Read the model definition and answer for the solid it produces. Units are mm, in the model's axes. A direction names the side the tool comes from. Round coordinates to 2 decimals unless told otherwise and drop trailing zeros. Write each loop counter-clockwise with the first axis right and the second up, starting at its lowest first coordinate (ties: lowest second). Pieces come first, ordered by that corner, then holes. Notation, with made-up numbers: (51, 62) - (87, 62) arc R21 cw to (87, 80) - close; hole circle Ø5 at (-9, 51). An arc over 180 degrees is marked (long way). Answer as CSV lines item,"result". Start each with the question number.
1) Find section A-A on z = 15.5. Determine the outline of the cut face in (x, y) (3 decimals), then the cut area to 3 significant figures.
2) Find section D-D on y = -2.5. Determine the outline of the cut face in (x, z), then the cut area to 3 significant figures.
3) For a pull along Y with two mould halves and no side action, classify faces 3 (the flat face through (6, -0.3, 2)), 4 (the flat face through (6, 15.2, 4)), 5 (the flat face through (11.5, 6, 2)), 6 (the flat face through (5, 5, 21.7)) as +Y half, -Y half, draft (parallel to the pull), parting line (faces both ways), or undercut.
4) Find section B-B on x = 3.25. Determine the outline of the cut face in (y, z).
5) Which of the six approach directions +Z, -Z, +X, -X, +Y, -Y give full straight-line access (tool end or side, diameter ignored) to faces 1 (the flat face through (-4, 6, 3)), 2 (the flat face through (-0.3, 6, 2))?
6) Consider line 1 along X through (y, z) = (4.5, 14); line 2 along Y through (x, z) = (12.25, -9.5). Determine where each line is inside the solid, lowest interval first.
from build123d import *

# Parameters (mm, degrees)
SKETCH1_W           = 19.2
SKETCH1_H           = 36.7
BOSS_EXTRUDE1_DEPTH = 19.2
SKETCH2_W           = 11.8
SKETCH2_H           = 11.8
CUT_EXTRUDE1_DEPTH  = 34.2
FILLET1_R           = 3.175


with BuildPart() as part:
    # Sketch1 → Boss-Extrude1 (new body)
    with BuildSketch(Plane.XZ.offset(4)):
        with Locations((5.6, 3.35)):
            Rectangle(SKETCH1_W, SKETCH1_H)
    extrude(amount=-BOSS_EXTRUDE1_DEPTH)

    # Sketch2 → Cut-Extrude1 (cut)
    with BuildSketch(Plane(origin=(0, 0, -15), x_dir=(-1, 0, 0), z_dir=(0, 0, -1))):
        with Locations((-5.6, 5.6)):
            Rectangle(SKETCH2_W, SKETCH2_H)
    extrude(amount=-CUT_EXTRUDE1_DEPTH, mode=Mode.SUBTRACT)

    # Fillet1
    fillet1_edges = [part.edges().sort_by_distance(p)[0] for p in [
        (-4, 15.2, 3.35),
        (15.2, 15.2, 3.35),
        (-4, -4, 3.35),
        (15.2, -4, 3.35),
    ]]
    fillet(fillet1_edges, radius=FILLET1_R)


solid = part.part
Check values:
1,outline,"(-4, -0.825) arc R3.175 ccw to (-0.825, -4) - (12.025, -4) arc R3.175 ccw to (15.2, -0.825) - (15.2, 12.025) arc R3.175 ccw to (12.025, 15.2) - (-0.825, 15.2) arc R3.175 ccw to (-4, 12.025) - close; hole (-0.3, -0.3) - (11.5, -0.3) - (11.5, 11.5) - (-0.3, 11.5) - close"
1,area,"221 mm^2"
2,outline,"(-3.52, -15) - (14.72, -15) - (14.72, 21.7) - (-3.52, 21.7) - close"
2,area,"670 mm^2"
3,face 3,"undercut"
3,face 4,"+Y half"
3,face 5,"undercut"
3,face 6,"draft"
4,outline,"(-4, -15) - (-0.3, -15) - (-0.3, 19.2) - (11.5, 19.2) - (11.5, -15) - (15.2, -15) - (15.2, 21.7) - (-4, 21.7) - close"
5,face 1,"+Z, -Z, -X, +Y, -Y"
5,face 2,"-Z"
6,line 1,"x = -4 to -0.3, 11.5 to 15.2"
6,line 2,"y = -3.99 to 15.19"
